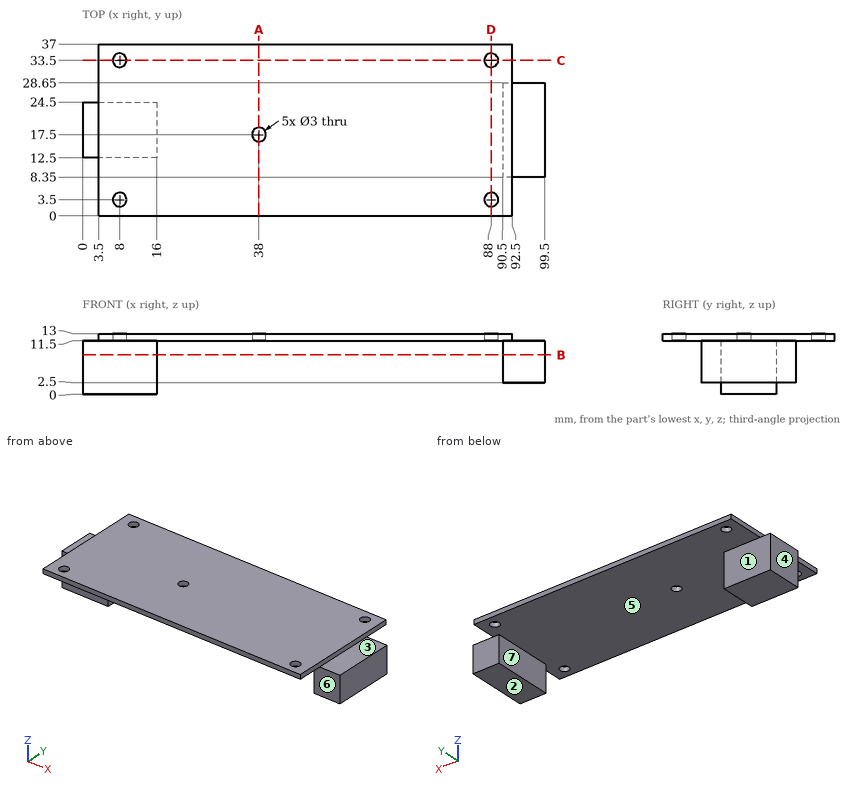
Can you work these out from the drawing? Everything is in mm from the part's minimum corner. A direction names the side the tool comes from. Give positions to 0.01 mm unless a question says otherwise; leave off trailing zeros. Order: outer loops, then holes, each group sorted by start corner. A loop starts at its lowest first (then second) coordinate and runs counter-clockwise, first axis right, second up.
1. For the marked faces 1, 2 and 3, which set-ups out of +Z, -Z, +X, -X, +Y, -Y let a thin tool reach every point of the face, with its end or its side?
2. I need wall thicknesses on L1, parallel to Y at x = 8, z = 12.65; L2, parallel to X at y = 16, z = 5.5; L3, parallel to Z at x = 70.5, y = 34.5. Which ranges of each line are inside material? Lowest first, please.
3. Suppose I cut it at B-B (z = 8.5). List the corners of the cut face in (x, y) for me, plus the area to 3 significant figures.
4. Suppose I cut it at D-D (x = 88). List the corners of the cut face in (y, z) for me.
5. Will these pins go through, and if not, where does the flat tip stop? P1, Ø10, axis at x = 93, y = 19, coming from the -Z side; P2, Ø5, axis at x = 8, y = 33.5, coming from the -Z side; P3, Ø7, axis at x = 95, z = 5.5, coming from the +Y side; P4, Ø7, axis at x = 94, z = 8.5, coming from the -Y side.
6. Suppose I cut it at A-A (x = 38). List the corners of the cut face in (y, z) for me, plus the area to 3 significant figures.
7. We'd pull the mould along X, two halves only. Please class the marked faces 4, 5, 6 and 7: pulls with the +X half, pulls with the -X half, needs draft (parallel to the pull), parting line crosses it, or undercut.
8. Suppose I cut it at C-C (y = 33.5). List the corners of the cut face in (x, z) for me.
Solved:
1. face 1: -Z, -X, +Y
1. face 2: -Z, +X, +Y, -Y
1. face 3: +Z, +X, +Y, -Y
2. L1: y = 0 to 2, 5 to 32, 35 to 37
2. L2: x = 0 to 16, 90.5 to 99.5
2. L3: z = 11.5 to 13
3. outline: (0, 12.5) - (16, 12.5) - (16, 24.5) - (0, 24.5) - close; (90.5, 8.35) - (99.5, 8.35) - (99.5, 28.65) - (90.5, 28.65) - close
3. area: 375 mm2
4. outline: (0, 11.5) - (2, 11.5) - (2, 13) - (0, 13) - close; (5, 11.5) - (32, 11.5) - (32, 13) - (5, 13) - close; (35, 11.5) - (37, 11.5) - (37, 13) - (35, 13) - close
5. P1: stops at z = 2.5
5. P2: stops at z = 11.5
5. P3: stops at y = 28.65
5. P4: stops at y = 0
6. outline: (0, 11.5) - (16, 11.5) - (16, 13) - (0, 13) - close; (19, 11.5) - (37, 11.5) - (37, 13) - (19, 13) - close
6. area: 51.0 mm2
7. face 4: pulls with the -X half
7. face 5: undercut
7. face 6: needs draft
7. face 7: undercut
8. outline: (3.5, 11.5) - (6.5, 11.5) - (6.5, 13) - (3.5, 13) - close; (9.5, 11.5) - (86.5, 11.5) - (86.5, 13) - (9.5, 13) - close; (89.5, 11.5) - (92.5, 11.5) - (92.5, 13) - (89.5, 13) - close
